from build123d import *

# Parameters (mm, degrees)
F0_W     = 2008.886
F0_H     = 119.888
F1_DEPTH = 1044.956
F2_W     = 738.8298484659
F2_H     = 75.2589369982
F2_W_2   = 726.7765416155
F3_DEPTH = 1044.956
F4_W     = 406.4
F4_H     = 81.788
F5_DEPTH = 2008.886


with BuildPart() as f1:
    # F0 (on Front) → F1 (new body)
    with BuildSketch(Plane.XZ):
        with Locations((433.0359270411, -67.1071302024)):
            Rectangle(F0_W, F0_H)
    extrude(amount=F1_DEPTH)

    # F2 (on face) → F3 (cut)
    with BuildSketch(Plane(origin=(0, 0, 0), x_dir=(-1, 0, 0), z_dir=(0, 1, 0))):
        with Locations((74.992148726, -89.4216617033)):
            Rectangle(F2_W, F2_H)
        with Locations((-947.0906562333, -89.4216617033)):
            Rectangle(F2_W_2, F2_H)
    extrude(amount=-F3_DEPTH, mode=Mode.SUBTRACT)

    # F4 (on face) → F5 (cut)
    with BuildSketch(Plane(origin=(-571.4070729589, 0, 0), x_dir=(0, -1, 0), z_dir=(-1, 0, 0))):
        with Locations((254, -73.4571302024)):
            Rectangle(F4_W, F4_H)
        with Locations((790.956, -73.4571302024)):
            Rectangle(F4_W, F4_H)
    extrude(amount=-F5_DEPTH, mode=Mode.SUBTRACT)


solid = f1.part
Verification items for the finished model (mm, model axes). A direction names the side the tool comes from. Give positions to 0.01 mm unless a question says otherwise; leave off trailing zeros. Order: outer loops, then holes, each group sorted by start corner. A loop starts at its lowest first (then second) coordinate and runs counter-clockwise, first axis right, second up. Notation, with made-up numbers: M -17.5,69.5 L 35.5,69.5 A19 ccw 35.5,82.5 Z; hole C 86.25,66 d3. An arc over 180 degrees is marked long. Use one line per item in the form item = value. Start each with the question number.
Q1. Scan lines: line 1 along X through (y, z) = (-42, -60.5); line 2 along Y through (x, z) = (402.5, -90.5); line 3 along Z through (x, y) = (505.5, -880.5). Record each from-to range of solid material in increasing order. Write a range as [from, to].
Q2. Section check B-B (y = -378). Enter the section's corners in (x, z), then the cut area to 3 significant figures.
Q3. Access from +Z, -Z, +X, -X, +Y, -Y to the whole of each face (thin tool, end or side, straight path). Record for faces 4 (the flat face through (952, -25, -51.792)), 5 (the flat face through (437, -251, -114.351)), 6 (the flat face through (419, -515, -7.163)).
Q4. Section check C-C (y = -501). Enter the section's corners in (x, z).
Q5. Section check A-A (x = 318). Enter the section's corners in (y, z).
Q6. Mould release check, pull along X, two halves, no side actions. Record for faces 1 (the flat face through (-571.407, -399, -28)), 2 (the flat face through (419, -251, -32.563)), 3 (the flat face through (952, -1019, -51.792)): +X half, -X half, draft (parallel to the pull), parting line (faces both ways), or undercut.
Q7. Section check D-D (x = 1122). Enter the section's corners in (y, z).
Q8. Go/stop test with flat-tipped pins: pin 1 Ø5 at (x, y) = (41.5, -137) entering from -Z; pin 2 Ø15 at (x, y) = (-259, -1028) entering from -Z; pin 3 Ø24.5 at (x, z) = (145, -65.5) entering from +Y. Record where each tip stops, or that it passes through.
Evaluation:
q1.line_1 = [-571.41, -444.41], [294.42, 583.7], [1310.48, 1437.48]
q1.line_2 = [-1044.96, -994.16], [-587.76, -457.2], [-50.8, 0]
q1.line_3 = [-127.05, -114.35], [-32.56, -7.16]
q2.outline = M -571.41,-127.05 L -444.41,-127.05 L -444.41,-114.35 L -571.41,-114.35 Z; M -571.41,-32.56 L 1437.48,-32.56 L 1437.48,-7.16 L -571.41,-7.16 Z; M 294.42,-127.05 L 583.7,-127.05 L 583.7,-114.35 L 294.42,-114.35 Z; M 1310.48,-127.05 L 1437.48,-127.05 L 1437.48,-114.35 L 1310.48,-114.35 Z
q2.area = 57,900 mm2
q3.face_4 = -Z, +Y, -Y
q3.face_5 = +X, -X
q3.face_6 = +Z, +X, -X, +Y, -Y
q4.outline = M -571.41,-127.05 L -444.41,-127.05 L -444.41,-51.79 L 294.42,-51.79 L 294.42,-127.05 L 583.7,-127.05 L 583.7,-51.79 L 1310.48,-51.79 L 1310.48,-127.05 L 1437.48,-127.05 L 1437.48,-7.16 L -571.41,-7.16 Z
q5.outline = M -1044.96,-127.05 L 0,-127.05 L 0,-7.16 L -1044.96,-7.16 Z; hole M -994.16,-114.35 L -587.76,-114.35 L -587.76,-32.56 L -994.16,-32.56 Z; hole M -457.2,-114.35 L -50.8,-114.35 L -50.8,-32.56 L -457.2,-32.56 Z
q6.face_1 = -X half
q6.face_2 = draft
q6.face_3 = undercut
q7.outline = M -1044.96,-51.79 L -994.16,-51.79 L -994.16,-32.56 L -587.76,-32.56 L -587.76,-51.79 L -457.2,-51.79 L -457.2,-32.56 L -50.8,-32.56 L -50.8,-51.79 L 0,-51.79 L 0,-7.16 L -1044.96,-7.16 Z
q8.pin_1 = -32.56
q8.pin_2 = -51.79
q8.pin_3 = through
